from build123d import *

# Parameters (mm, degrees)
BOSS_EXTRUDE1_DEPTH = 10
BOSS_EXTRUDE2_DEPTH = 15
BOSS_EXTRUDE3_DEPTH = 10
CUT_EXTRUDE1_DEPTH  = 2.5
SKETCH5_R           = 1.5
CUT_EXTRUDE2_DEPTH  = 3
CUT_EXTRUDE3_START  = -2
SKETCH6_R           = 16
SKETCH6_R_2         = 1.5
CUT_EXTRUDE3_DEPTH  = 2
SKETCH7_R           = 10
BOSS_EXTRUDE4_DEPTH = 2.3
SKETCH8_R           = 2.5
BOSS_EXTRUDE5_DEPTH = 23


with BuildPart() as part:
    # Sketch1 → Boss-Extrude1 (new body)
    with BuildSketch(Plane(origin=(0, 0, 0), x_dir=(1, 0, 0), z_dir=(0, 1, 0))):
        Polygon((-17.464466094, 21), (17.464466094, 21), (21, 17.464466094), (21, -17.464466094), (17.464466094, -21), (-17.464466094, -21), (-21, -17.464466094), (-21, 17.464466094), align=None)
    extrude(amount=BOSS_EXTRUDE1_DEPTH)

    # Sketch2 → Boss-Extrude2 (add)
    with BuildSketch(Plane(origin=(0, 10, 0), x_dir=(1, 0, 0), z_dir=(0, 1, 0))):
        Polygon((-13.5, 21), (13.5, 21), (21, 13.5), (21, -13.5), (13.5, -21), (-13.5, -21), (-21, -13.5), (-21, 13.5), align=None)
    extrude(amount=BOSS_EXTRUDE2_DEPTH)

    # Sketch3 → Boss-Extrude3 (add)
    with BuildSketch(Plane(origin=(0, 25, 0), x_dir=(1, 0, 0), z_dir=(0, 1, 0))):
        Polygon((-17.464466094, 21), (17.464466094, 21), (21, 17.464466094), (21, -17.464466094), (17.464466094, -21), (-17.464466094, -21), (-21, -17.464466094), (-21, 17.464466094), align=None)
    extrude(amount=BOSS_EXTRUDE3_DEPTH)

    # Sketch4 → Cut-Extrude1 (cut)
    with BuildSketch(Plane(origin=(0, 35, 0), x_dir=(1, 0, 0), z_dir=(0, 1, 0))):
        Polygon((-12, 12), (-21, 12), (-21, 17.464466094), (-17.464466094, 21), (-12, 21), align=None)
        Polygon((12, 21), (12, 12), (21, 12), (21, 17.464466094), (17.464466094, 21), align=None)
        Polygon((12, -12), (21, -12), (21, -17.464466094), (17.464466094, -21), (12, -21), align=None)
        Polygon((-12, -21), (-12, -12), (-21, -12), (-21, -17.464466094), (-17.464466094, -21), align=None)
    extrude(amount=-CUT_EXTRUDE1_DEPTH, mode=Mode.SUBTRACT)

    # Sketch5 → Cut-Extrude2 (cut)
    with BuildSketch(Plane(origin=(0, 32.5, 0), x_dir=(1, 0, 0), z_dir=(0, 1, 0))):
        with Locations(Location((16.403805922, 16.403805922, 0), (0, 0, 270))):
            Circle(SKETCH5_R)
        with Locations(Location((-16.403805922, 16.403805922, 0), (0, 0, 90))):
            Circle(SKETCH5_R)
        with Locations(Location((-16.403805922, -16.403805922, 0), (0, 0, 270))):
            Circle(SKETCH5_R)
        with Locations(Location((16.403805922, -16.403805922, 0), (0, 0, 90))):
            Circle(SKETCH5_R)
    extrude(amount=-CUT_EXTRUDE2_DEPTH, mode=Mode.SUBTRACT)

    # Sketch6 → Cut-Extrude3 (cut)
    with BuildSketch(Plane.XZ.offset(CUT_EXTRUDE3_START)):
        with Locations(Location((0, 0, 0), (0, 0, 270))):
            Circle(SKETCH6_R)
        with Locations(Location((-16.403805922, -16.403805922, 0), (0, 0, 270))):
            Circle(SKETCH6_R_2)
        with Locations(Location((16.403805922, -16.403805922, 0), (0, 0, 90))):
            Circle(SKETCH6_R_2)
        with Locations(Location((-16.403805922, 16.403805922, 0), (0, 0, 90))):
            Circle(SKETCH6_R_2)
        with Locations(Location((16.403805922, 16.403805922, 0), (0, 0, 270))):
            Circle(SKETCH6_R_2)
    extrude(amount=CUT_EXTRUDE3_DEPTH, mode=Mode.SUBTRACT)

    # Sketch7 → Boss-Extrude4 (add)
    with BuildSketch(Plane.XZ.offset(-2)):
        with Locations(Location((0, 0, 0), (0, 0, 270))):
            Circle(SKETCH7_R)
    extrude(amount=BOSS_EXTRUDE4_DEPTH)

    # Sketch8 → Boss-Extrude5 (add)
    with BuildSketch(Plane.XZ.offset(0.3)):
        with Locations(Location((0, 0, 0), (0, 0, 270))):
            Circle(SKETCH8_R)
    extrude(amount=BOSS_EXTRUDE5_DEPTH)


solid = part.part
Geometry check sheet. Reference: the model listing, model coordinates, mm. A direction names the side the tool comes from. Give positions to 0.01 mm unless a question says otherwise; leave off trailing zeros. Write each loop counter-clockwise with the first axis right and the second up, starting at its lowest first coordinate (ties: lowest second). Pieces come first, ordered by that corner, then holes. Notation, with made-up numbers: M 26,85.25 L 80,85.25 A22 cw 80,110.25 Z; hole C 24.5,21 d2. An arc over 180 degrees is marked long. Answer as CSV lines item,"result". Start each with the question number.
Q1. Section check D-D, the plane z = 6.5. Record the cut outline in (x, y).
Q2. Tool access check on faces 4 (the face through (16, 29.5, 16)), 5 (the face through (18, 25, 18)), 6 (the face through (-17.3, 17.4, -17.2)), 7 (the face through (-10.4, 2, 0.2)). Record the directions out of +Z, -Z, +X, -X, +Y, -Y that give a thin tool (end or side, any length) a straight path to the whole face; none if there is none.
Q3. Release check for a two-part mould opening along Z. For faces 1 (the face through (19.257, 28.697, 19.207)), 2 (the face through (-15.14, 1.01, -17.21)), 3 (the face through (18, 10, -18)) record: pulls with the +Z half, pulls with the -Z half, needs draft (parallel to the pull), parting line crosses it, or undercut.
Q4. Section check C-C, the plane z = 0. Record the cut outline in (x, y).
Q5. Material ranges on L1, parallel to X at y = 1, z = 2; L2, parallel to Y at x = 6.5, z = 7; L3, parallel to Y at x = 10, z = 13.5, recorded low to high.
Q6. Section check A-A, the plane x = 0. Record the cut outline in (y, z), then the cut area to 3 significant figures.
Q7. Section check B-B, the plane y = 22.5. Record the cut outline in (x, z).
Q8. Go/stop test with flat-tipped pins: pin 1 (7 mm diameter, centred on x = -17, z = 16.5, fed in from +Y); pin 2 (2.5 mm diameter, centred on x = -16.4, z = 16.4, fed in from -Y); pin 3 (0.8 mm diameter, centred on y = 34, z = 14.5, fed in from +X). Record where each tip stops, or that it passes through.
Geometry says:
1,outline,"M -21,0 L -14.62,0 L -14.62,2 L -7.6,2 L -7.6,-0.3 L 7.6,-0.3 L 7.6,2 L 14.62,2 L 14.62,0 L 21,0 L 21,35 L -21,35 Z"
2,face 4,"+Y"
2,face 5,"+Z, +X"
2,face 6,"-Z, -X"
2,face 7,"-Y"
3,face 1,"pulls with the +Z half"
3,face 2,"undercut"
3,face 3,"needs draft"
4,outline,"M -21,0 L -16,0 L -16,2 L -10,2 L -10,-0.3 L -2.5,-0.3 L -2.5,-23.3 L 2.5,-23.3 L 2.5,-0.3 L 10,-0.3 L 10,2 L 16,2 L 16,0 L 21,0 L 21,35 L -21,35 Z"
5,L1,"-21 to -15.87, -9.8 to 9.8, 15.87 to 21"
5,L2,"-0.3 to 35"
5,L3,"0 to 35"
6,outline,"M -23.3,-2.5 L -0.3,-2.5 L -0.3,-10 L 2,-10 L 2,-16 L 0,-16 L 0,-21 L 35,-21 L 35,21 L 0,21 L 0,16 L 2,16 L 2,10 L -0.3,10 L -0.3,2.5 L -23.3,2.5 Z"
6,area,"1,570 mm^2"
7,outline,"M -21,-13.5 L -13.5,-21 L 13.5,-21 L 21,-13.5 L 21,13.5 L 13.5,21 L -13.5,21 L -21,13.5 Z"
8,pin 1,"y = 32.5"
8,pin 2,"y = 2"
8,pin 3,"x = 12"
